from build123d import *

# Parameters (mm, degrees)
CROQUIS2_R              = 0.5
CROQUIS2_R_2            = 1.5
CROQUIS2_W              = 1.8
CROQUIS2_H              = 4
CROQUIS2_W_2            = 9
CROQUIS2_H_2            = 3
CROQUIS2_W_3            = 9.7
CROQUIS2_H_3            = 2.94
CROQUIS2_W_4            = 10.628979849
CROQUIS2_H_4            = 6
SALIENTE_EXTRUIR1_DEPTH = 3


with BuildPart() as part:
    # Croquis2 → Saliente-Extruir1 (new body)
    with BuildSketch(Plane.XY):
        with BuildLine():
            Line((33708.140369107, 12866.76836421), (33708.140369107, 12884.268432106))
            Line((33708.140369107, 12884.268432106), (33710.140369103, 12884.268296333))
            ThreePointArc((33710.140369103, 12884.268296333), (33714.140640639, 12888.268024778), (33710.140912194, 12892.268296314))
            Line((33710.140912194, 12892.268296314), (33708.14091219, 12892.268296314))
            Line((33708.14091219, 12892.268296314), (33708.140369107, 12909.76836421))
            Line((33708.140369107, 12909.76836421), (33711.140369107, 12909.76836421))
            Line((33711.140369107, 12909.76836421), (33711.140369107, 12920.76836421))
            Line((33711.140369107, 12920.76836421), (33699.140369107, 12920.76836421))
            Line((33699.140369107, 12920.76836421), (33699.140369107, 12923.76836421))
            Line((33699.140369107, 12923.76836421), (33689.140369107, 12923.76836421))
            Line((33689.140369107, 12923.76836421), (33689.140369107, 12920.76836421))
            Line((33689.140369107, 12920.76836421), (33679.140369107, 12920.76836421))
            Line((33679.140369107, 12920.76836421), (33679.140369107, 12923.76836421))
            Line((33679.140369107, 12923.76836421), (33669.140369107, 12923.76836421))
            Line((33669.140369107, 12923.76836421), (33669.140369107, 12920.76836421))
            Line((33669.140369107, 12920.76836421), (33649.140369107, 12920.76836421))
            Line((33649.140369107, 12920.76836421), (33649.140369107, 12923.76836421))
            ThreePointArc((33649.140369107, 12923.76836421), (33648.261689451, 12925.889684554), (33646.140369107, 12926.76836421))
            Line((33646.140369107, 12926.76836421), (33622.140369107, 12926.76836421))
            ThreePointArc((33622.140369107, 12926.76836421), (33620.019048764, 12925.889684554), (33619.140369107, 12923.76836421))
            Line((33619.140369107, 12923.76836421), (33619.140369107, 12920.76836421))
            Line((33619.140369107, 12920.76836421), (33599.140369107, 12920.76836421))
            Line((33599.140369107, 12920.76836421), (33599.140369107, 12923.76836421))
            Line((33599.140369107, 12923.76836421), (33589.140369107, 12923.76836421))
            Line((33589.140369107, 12923.76836421), (33589.140369107, 12920.76836421))
            Line((33589.140369107, 12920.76836421), (33579.140369107, 12920.76836421))
            Line((33579.140369107, 12920.76836421), (33579.140369107, 12923.76836421))
            Line((33579.140369107, 12923.76836421), (33569.140369107, 12923.76836421))
            Line((33569.140369107, 12923.76836421), (33569.140369107, 12920.76836421))
            Line((33569.140369107, 12920.76836421), (33557.140369107, 12920.76836421))
            Line((33557.140369107, 12920.76836421), (33557.140369107, 12909.76836421))
            Line((33557.140369107, 12909.76836421), (33560.140369107, 12909.76836421))
            Line((33560.140369107, 12909.76836421), (33560.139826016, 12892.268432087))
            Line((33560.139826016, 12892.268432087), (33558.13982602, 12892.268296314))
            ThreePointArc((33558.13982602, 12892.268296314), (33554.140097575, 12888.268024778), (33558.140369112, 12884.268296333))
            Line((33558.140369112, 12884.268296333), (33560.140369107, 12884.268432106))
            Line((33560.140369107, 12884.268432106), (33560.140369107, 12866.76836421))
            Line((33560.140369107, 12866.76836421), (33559.115527824, 12866.76836421))
            Line((33559.115527824, 12866.76836421), (33558.815527824, 12866.76836421))
            Line((33558.815527824, 12866.76836421), (33557.140369107, 12866.76836421))
            Line((33557.140369107, 12866.76836421), (33557.140369107, 12861.352876793))
            Line((33557.140369107, 12861.352876793), (33557.140369107, 12861.058331403))
            Line((33557.140369107, 12861.058331403), (33557.140369107, 12855.76836421))
            Line((33557.140369107, 12855.76836421), (33569.140369107, 12855.76836421))
            Line((33569.140369107, 12855.76836421), (33569.140369107, 12852.76836421))
            Line((33569.140369107, 12852.76836421), (33579.140369107, 12852.76836421))
            Line((33579.140369107, 12852.76836421), (33579.140369107, 12855.76836421))
            Line((33579.140369107, 12855.76836421), (33589.140369107, 12855.76836421))
            Line((33589.140369107, 12855.76836421), (33589.140369107, 12852.76836421))
            Line((33589.140369107, 12852.76836421), (33599.140369107, 12852.76836421))
            Line((33599.140369107, 12852.76836421), (33599.140369107, 12855.76836421))
            Line((33599.140369107, 12855.76836421), (33609.140369107, 12855.76836421))
            Line((33609.140369107, 12855.76836421), (33619.140369107, 12855.76836421))
            Line((33619.140369107, 12855.76836421), (33619.140369107, 12852.76836421))
            ThreePointArc((33619.140369107, 12852.76836421), (33620.019048764, 12850.647043866), (33622.140369107, 12849.76836421))
            Line((33622.140369107, 12849.76836421), (33646.140369107, 12849.76836421))
            ThreePointArc((33646.140369107, 12849.76836421), (33648.261689451, 12850.647043866), (33649.140369107, 12852.76836421))
            Line((33649.140369107, 12852.76836421), (33649.140369107, 12855.76836421))
            Line((33649.140369107, 12855.76836421), (33659.140369107, 12855.76836421))
            Line((33659.140369107, 12855.76836421), (33665.009331237, 12855.76836421))
            Line((33665.009331237, 12855.76836421), (33665.309331237, 12855.76836421))
            Line((33665.309331237, 12855.76836421), (33669.140369107, 12855.76836421))
            Line((33669.140369107, 12855.76836421), (33669.140369107, 12852.76836421))
            Line((33669.140369107, 12852.76836421), (33679.140369107, 12852.76836421))
            Line((33679.140369107, 12852.76836421), (33679.140369107, 12855.76836421))
            Line((33679.140369107, 12855.76836421), (33685.009331237, 12855.76836421))
            Line((33685.009331237, 12855.76836421), (33685.309331237, 12855.76836421))
            Line((33685.309331237, 12855.76836421), (33689.140369107, 12855.76836421))
            Line((33689.140369107, 12855.76836421), (33689.140369107, 12852.76836421))
            Line((33689.140369107, 12852.76836421), (33699.140369107, 12852.76836421))
            Line((33699.140369107, 12852.76836421), (33699.140369107, 12855.76836421))
            Line((33699.140369107, 12855.76836421), (33711.140369107, 12855.76836421))
            Line((33711.140369107, 12855.76836421), (33711.140369107, 12866.76836421))
            Line((33711.140369107, 12866.76836421), (33708.140369107, 12866.76836421))
        make_face()
        with Locations((33641.140369107, 12899.76836421)):
            Circle(CROQUIS2_R, mode=Mode.SUBTRACT)
        with Locations((33641.140369107, 12878.76836421)):
            Circle(CROQUIS2_R, mode=Mode.SUBTRACT)
        with Locations((33680.011779321, 12890.673818632)):
            Circle(CROQUIS2_R_2, mode=Mode.SUBTRACT)
        with Locations((33588.287365241, 12890.673818632)):
            Circle(CROQUIS2_R_2, mode=Mode.SUBTRACT)
        with Locations((33611.040369107, 12889.26836421)):
            Circle(CROQUIS2_R, mode=Mode.SUBTRACT)
        with Locations((33709.140640651, 12888.26836421)):
            Circle(CROQUIS2_R_2, mode=Mode.SUBTRACT)
        with Locations((33559.140097564, 12888.26836421)):
            Circle(CROQUIS2_R_2, mode=Mode.SUBTRACT)
        with Locations((33634.140369107, 12922.26836421)):
            Circle(CROQUIS2_R_2, mode=Mode.SUBTRACT)
        with Locations((33634.140369107, 12854.26836421)):
            Circle(CROQUIS2_R_2, mode=Mode.SUBTRACT)
        Polygon((33589.787365241, 12868.173818632), (33586.787365241, 12868.173818632), (33586.687365241, 12868.173818632), (33586.687365241, 12878.173818632), (33586.787365241, 12878.173818632), (33589.787365241, 12878.173818632), (33589.887365241, 12878.173818632), (33589.887365241, 12868.173818632), align=None, mode=Mode.SUBTRACT)
        Polygon((33589.787365241, 12903.173818632), (33586.787365241, 12903.173818632), (33586.737365241, 12903.173818632), (33586.687365241, 12903.173818632), (33586.687365241, 12913.173818632), (33586.787365241, 12913.173818632), (33589.787365241, 12913.173818632), (33589.887365241, 12913.173818632), (33589.887365241, 12903.173818632), (33589.837365241, 12903.173818632), align=None, mode=Mode.SUBTRACT)
        Polygon((33681.493372973, 12868.173818632), (33678.493372973, 12868.173818632), (33678.393372973, 12868.173818632), (33678.393372973, 12878.173818632), (33678.493372973, 12878.173818632), (33681.493372973, 12878.173818632), (33681.593372973, 12878.173818632), (33681.593372973, 12868.173818632), align=None, mode=Mode.SUBTRACT)
        Polygon((33681.493372973, 12903.173818632), (33678.493372973, 12903.173818632), (33678.393372973, 12903.173818632), (33678.393372973, 12913.173818632), (33678.493372973, 12913.173818632), (33681.493372973, 12913.173818632), (33681.593372973, 12913.173818632), (33681.593372973, 12903.173818632), align=None, mode=Mode.SUBTRACT)
        with Locations((33564.890369107, 12909.90336421)):
            Rectangle(CROQUIS2_W, CROQUIS2_H, mode=Mode.SUBTRACT)
        with Locations((33573.390369107, 12909.90336421)):
            Rectangle(CROQUIS2_W, CROQUIS2_H, mode=Mode.SUBTRACT)
        with Locations((33564.890369107, 12888.14336421)):
            Rectangle(CROQUIS2_W, CROQUIS2_H, mode=Mode.SUBTRACT)
        with Locations((33573.390369107, 12888.14336421)):
            Rectangle(CROQUIS2_W, CROQUIS2_H, mode=Mode.SUBTRACT)
        with Locations((33564.890369107, 12866.38336421)):
            Rectangle(CROQUIS2_W, CROQUIS2_H, mode=Mode.SUBTRACT)
        with Locations((33573.390369107, 12866.38336421)):
            Rectangle(CROQUIS2_W, CROQUIS2_H, mode=Mode.SUBTRACT)
        with Locations((33600.540369107, 12877.26836421)):
            Rectangle(CROQUIS2_W_2, CROQUIS2_H_2, mode=Mode.SUBTRACT)
        with Locations((33619.140369107, 12861.26836421)):
            Rectangle(CROQUIS2_W_3, CROQUIS2_H_3, mode=Mode.SUBTRACT)
        with Locations((33633.931190824, 12868.26836421)):
            Rectangle(CROQUIS2_W_4, CROQUIS2_H_4, mode=Mode.SUBTRACT)
        with Locations((33629.890369107, 12888.14336421)):
            Rectangle(CROQUIS2_W, CROQUIS2_H, mode=Mode.SUBTRACT)
        with Locations((33638.390369107, 12888.14336421)):
            Rectangle(CROQUIS2_W, CROQUIS2_H, mode=Mode.SUBTRACT)
        with Locations((33638.390369107, 12909.90336421)):
            Rectangle(CROQUIS2_W, CROQUIS2_H, mode=Mode.SUBTRACT)
        with Locations((33629.890369107, 12909.90336421)):
            Rectangle(CROQUIS2_W, CROQUIS2_H, mode=Mode.SUBTRACT)
        with Locations((33649.140369107, 12861.26836421)):
            Rectangle(CROQUIS2_W_3, CROQUIS2_H_3, mode=Mode.SUBTRACT)
        with Locations((33667.740369107, 12877.26836421)):
            Rectangle(CROQUIS2_W_2, CROQUIS2_H_2, mode=Mode.SUBTRACT)
        with Locations((33694.890369107, 12909.90336421)):
            Rectangle(CROQUIS2_W, CROQUIS2_H, mode=Mode.SUBTRACT)
        with Locations((33703.390369107, 12909.90336421)):
            Rectangle(CROQUIS2_W, CROQUIS2_H, mode=Mode.SUBTRACT)
        with Locations((33694.890369107, 12888.14336421)):
            Rectangle(CROQUIS2_W, CROQUIS2_H, mode=Mode.SUBTRACT)
        with Locations((33703.390369107, 12888.14336421)):
            Rectangle(CROQUIS2_W, CROQUIS2_H, mode=Mode.SUBTRACT)
        with Locations((33694.890369107, 12866.38336421)):
            Rectangle(CROQUIS2_W, CROQUIS2_H, mode=Mode.SUBTRACT)
        with Locations((33703.390369107, 12866.38336421)):
            Rectangle(CROQUIS2_W, CROQUIS2_H, mode=Mode.SUBTRACT)
    extrude(amount=SALIENTE_EXTRUIR1_DEPTH)


solid = part.part
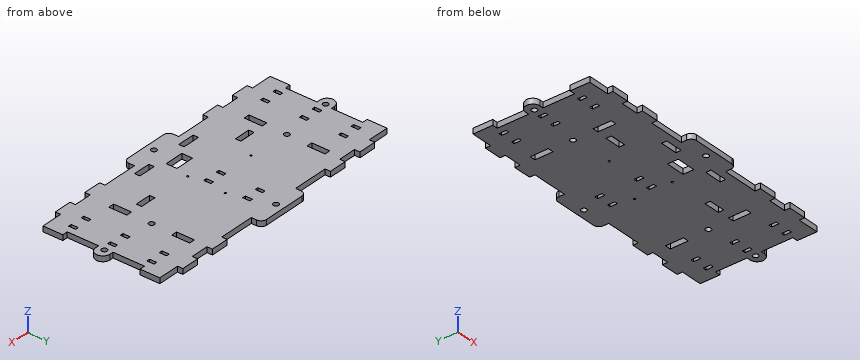
The listing builds one solid part. Answer for the finished solid, in the listing's coordinates (mm). Round coordinates to 2 decimals unless told otherwise and drop trailing zeros. Write each loop counter-clockwise with the first axis right and the second up, starting at its lowest first coordinate (ties: lowest second). Pieces come first, ordered by that corner, then holes. Notation, with made-up numbers: (87.25, 77.25) - (129.25, 77.25) arc R30 ccw to (129.25, 106.25) - close; hole circle Ø1 at (-1.75, 31). An arc over 180 degrees is marked (long way). Use a Markdown table: item, result. Add a question column.
1. Consider line 1 (X direction, y = 12868, z = 0.2); line 2 (X direction, y = 12906, z = 1.2); line 3 (X direction, y = 12869, z = 2.2). Determine where each line is inside the solid, lowest interval first.
2. The part is cut by section B-B (z = 1.2). Give the number of separate pieces and of enclosed holes in the cut face, and give its area (3 significant figures).
3. The part is cut by section A-A (y = 12917.5). Write down the section's boundary in (x, z), and give its area (3 significant figures).
4. Flat-ended cylindrical pins translate along their axes: P1, Ø0.9, axis at y = 12922, z = 2, coming from the +X side; P2, Ø1.5, axis at y = 12862, z = 1, coming from the -X side; P3, Ø1.5, axis at y = 12876.5, z = 1.5, coming from the +X side. Find the tip coordinate at first contact, or state that the pin passes through.
Reported:
| question | item | result |
|---|---|---|
| 1 | line 1 | 33560.14 to 33563.99, 33565.79 to 33572.49, 33574.29 to 33628.62, 33639.25 to 33693.99, 33695.79 to 33702.49, 33704.29 to 33708.14 |
| 1 | line 2 | 33560.14 to 33586.69, 33589.89 to 33678.39, 33681.59 to 33708.14 |
| 1 | line 3 | 33560.14 to 33586.69, 33589.89 to 33628.62, 33639.25 to 33678.39, 33681.59 to 33708.14 |
| 2 | separate pieces | 1 |
| 2 | enclosed holes | 34 |
| 2 | area | 9,960 mm^2 |
| 3 | outline | (33557.14, 0) - (33711.14, 0) - (33711.14, 3) - (33557.14, 3) - close |
| 3 | area | 462 mm^2 |
| 4 | P1 | x = 33699.14 |
| 4 | P2 | x = 33557.14 |
| 4 | P3 | x = 33708.14 |
